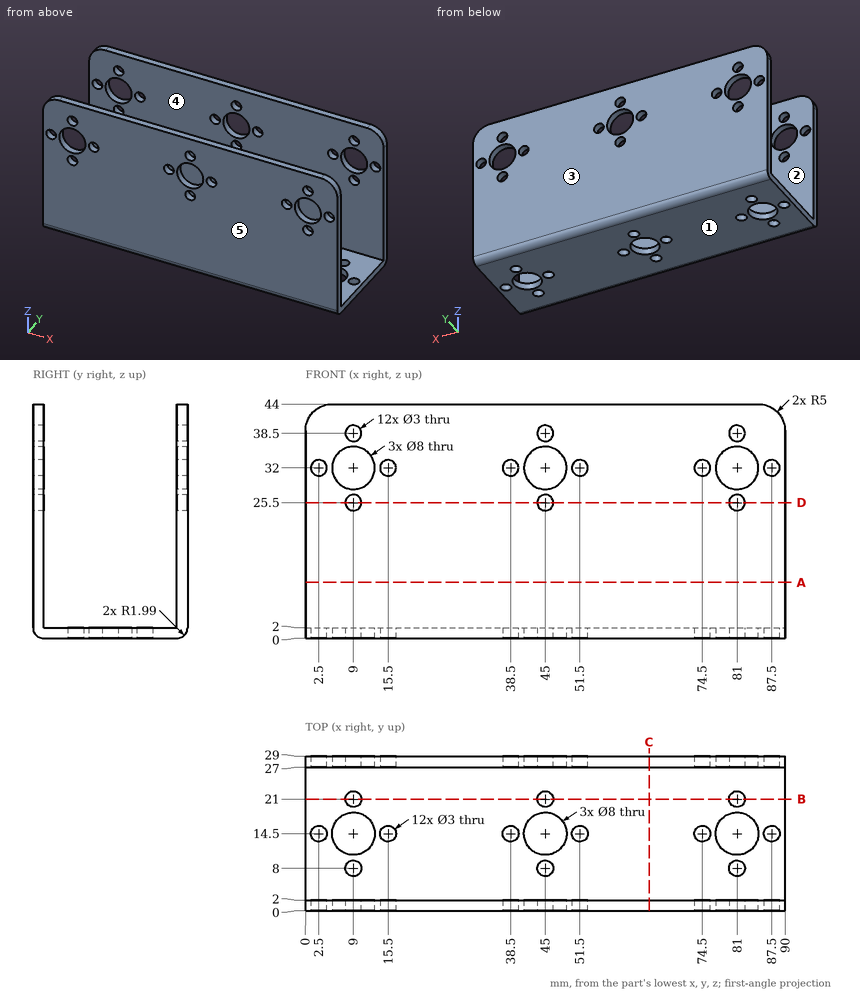
Here's the drawing with two shaded views (mm, measured from the low corner). I have some questions. A direction names the side the tool comes from. Give positions to 0.01 mm unless a question says otherwise; leave off trailing zeros. Loops run counter-clockwise (first coordinate to the right, second up) from the corner with the lowest first, then second, coordinate; pieces in that order, holes last. Notation, with made-up numbers: (-0.5, 88.5) - (26.5, 88.5) arc R29 cw to (26.5, 121.5) - close; hole circle Ø2 at (-8, -16). An arc over 180 degrees is marked (long way). One line per item, written item: value.
(1) I'm going to push flat-ended pins straight in: pin 1 (5 mm diameter, centred on x = 38.5, y = 14.5, fed in from +Z); pin 2 (2.5 mm diameter, centred on x = 81, z = 25.5, fed in from +Y). Where does each tip first touch, or does it pass through?
Verdict:
pin 1: z = 2
pin 2: through
(2) On a 3-axis mill with a long thin cutter (end or side, diameter ignored), from which of +Z, -Z, +X, -X, +Y, -Y can I reach the whole of each face in a straight line? I mean the marked faces 4 and 5. Say none if no direction works.
Verdict:
face 4: +Z, +X, -X
face 5: +Z, -Z, +X, -X, -Y
(3) I need wall thicknesses on line 1 along Y through (x, z) = (61, 16); line 2 along Z through (x, y) = (45, 1); line 3 along Y through (x, z) = (81, 1.1). Which ranges of each line are inside material? Lowest first, please.
Verdict:
line 1: 0 to 2, 27 to 29
line 2: 0.26 to 24, 27 to 28, 36 to 37, 40 to 44
line 3: 0.21 to 6.5, 9.5 to 10.5, 18.5 to 19.5, 22.5 to 28.79
(4) If we section it at A-A, the plane z = 10.5: List the corners of the cut face in (x, y) for me, plus the area to 3 significant figures.
Verdict:
outline: (0, 0) - (90, 0) - (90, 2) - (0, 2) - close; (0, 27) - (90, 27) - (90, 29) - (0, 29) - close
area: 360 mm^2
(5) If we section it at D-D, the plane z = 25.5: State how many separate pieces and enclosed holes the cut face has, plus the area to 3 significant figures.
Verdict:
separate pieces: 8
enclosed holes: 0
area: 324 mm^2
(6) If we mould it in two halves opening along Y, with no side actions, what happens to the marked faces 1, 2 and 3? For each: released by +Y, released by -Y, zero draft, split by the parting line, or undercut.
Verdict:
face 1: zero draft
face 2: undercut
face 3: released by +Y
(7) If we section it at C-C, the plane x = 64.5: List the corners of the cut face in (y, z) for me.
Verdict:
outline: (0, 1.99) arc R1.99 ccw to (1.99, 0) - (27.01, 0) arc R1.99 ccw to (29, 1.99) - (29, 44) - (27, 44) - (27, 2) - (2, 2) - (2, 44) - (0, 44) - close
(8) If we section it at B-B, the plane y = 21: List the corners of the cut face in (x, z) for me, plus the area to 3 significant figures.
Verdict:
outline: (0, 0) - (7.5, 0) - (7.5, 2) - (0, 2) - close; (10.5, 0) - (43.5, 0) - (43.5, 2) - (10.5, 2) - close; (46.5, 0) - (79.5, 0) - (79.5, 2) - (46.5, 2) - close; (82.5, 0) - (90, 0) - (90, 2) - (82.5, 2) - close
area: 162 mm^2
